Can you work these out from the model? Positions are in its coordinate system, mm. Face numbers are marked on the shaded views. A direction names the side the tool comes from. Coordinates: 2 decimals unless noted, no trailing zeros. Order: outer loops, then holes, each group sorted by start corner. A loop starts at its lowest first (then second) coordinate and runs counter-clockwise, first axis right, second up. Notation, with made-up numbers: (20.25, -25) -> (37.25, -25) arc R12 ccw to (37.25, -20) -> close; hole circle Ø6 at (-6, 37.5). An arc over 180 degrees is marked (long way). Return JSON: item names as keys, results as strings. Group by question number.
1) If we section it at D-D, the plane y = 0: Please give me the cut outline in (x, z).
2) For the marked faces 4, 5 and 6, which set-ups out of +Z, -Z, +X, -X, +Y, -Y let a thin tool reach every point of the face, with its end or its side?
3) If we section it at C-C, the plane z = -19.5: Please give me the cut outline in (x, y), then the cut area to 3 significant figures.
4) If we section it at A-A, the plane y = 23.5: Please give me the cut outline in (x, z).
5) Thinking about a two-plate mould opening in Z: for the marked faces 1, 2 and 3, which applies, +Z half, -Z half, draft (parallel to the pull), parting line (faces both ways), or undercut?
6) If we section it at B-B, the plane x = 0: Please give me the cut outline in (y, z), then the cut area to 3 significant figures.
7) If I drill on probe 1 along X at (y, z) = (22, -8); probe 2 along Y at (x, z) = (0, 1.7); probe 3 along Z at (x, y) = (0.25, 7.5), over which ranges is the centre line in solid material (lowest first)? Write a range as from..to.
8) For pin 1 (5.5 mm diameter, centred on y = 41.7, z = -19.5, fed in from -X); pin 2 (5 mm diameter, centred on x = 0, y = 0, fed in from -Z); pin 3 (4 mm diameter, centred on x = -3.5, z = -7, fed in from -Y), each with a flat end and sliding along its axis, tell me the tip position at first contact or that it passes through.
from build123d import *
from OCP.BRepFilletAPI import BRepFilletAPI_MakeChamfer

# Parameters (mm, degrees)
SKETCH1_W           = 18
SKETCH1_H           = 25.4
SKETCH1_R           = 3.25
BOSS_EXTRUDE1_DEPTH = 6
SKETCH2_W           = 18
SKETCH2_H           = 37.5
BOSS_EXTRUDE2_DEPTH = 6
SKETCH3_W           = 5.95
SKETCH3_H           = 37.5
BOSS_EXTRUDE3_DEPTH = 35
SKETCH4_R           = 2.15
CUT_EXTRUDE1_DEPTH  = 65.806944072
CUT_EXTRUDE2_REACH  = 66.807
SKETCH5_R           = 2.95
FILLET1_R           = 10
FILLET2_R           = 6
CHAMFER1_SIZE       = 1
CHAMFER1_SIZE2      = 1.732050808
CHAMFER2_SIZE       = 1
CHAMFER2_SIZE2      = 1.732050808
FILLET3_R           = 1


with BuildPart() as part:
    # Sketch1 → Boss-Extrude1 (new body)
    with BuildSketch(Plane.XY):
        Rectangle(SKETCH1_W, SKETCH1_H)
        Circle(SKETCH1_R, mode=Mode.SUBTRACT)
    boss_extrude1 = extrude(amount=BOSS_EXTRUDE1_DEPTH)

    # Sketch2 → Boss-Extrude2 (add)
    with BuildSketch(Plane(origin=(0, 12.7, 0), x_dir=(1, 0, 0), z_dir=(0, 1, 0))):
        with Locations((0, 12.75)):
            Rectangle(SKETCH2_W, SKETCH2_H)
    extrude(amount=BOSS_EXTRUDE2_DEPTH)

    # Mirror1: Boss-Extrude1 across plane
    add(boss_extrude1.mirror(Plane.XY.offset(-12.75)))

    # Sketch3 → Boss-Extrude3 (add)
    with BuildSketch(Plane(origin=(0, 18.7, 0), x_dir=(1, 0, 0), z_dir=(0, 1, 0))):
        with Locations((6.025, 12.75)):
            Rectangle(SKETCH3_W, SKETCH3_H)
    boss_extrude3 = extrude(amount=BOSS_EXTRUDE3_DEPTH)

    # Mirror2: Boss-Extrude3 across plane
    add(boss_extrude3.mirror(Plane(origin=(0, 0, 0), x_dir=(0, 0, 1), z_dir=(1, 0, 0))))

    # Sketch4 → Cut-Extrude1 (cut, through all)
    with BuildSketch(Plane(origin=(9, 0, 0), x_dir=(0, 0, -1), z_dir=(1, 0, 0))):
        with Locations((19.5, 41.7)):
            Circle(SKETCH4_R)
    extrude(amount=-CUT_EXTRUDE1_DEPTH, mode=Mode.SUBTRACT)

    # Sketch5 → Cut-Extrude2 (cut, up to next)
    with BuildSketch(Plane.ZY.offset(9), mode=Mode.PRIVATE) as cut_extrude2_sk1:
        with Locations((-19.5, 41.7)):
            Circle(SKETCH5_R)
    cut_extrude2_tool1 = extrude(cut_extrude2_sk1.sketch, amount=-CUT_EXTRUDE2_REACH, mode=Mode.PRIVATE) & part.part
    add(cut_extrude2_tool1.solids().sort_by_distance((-9, 41.7, -19.5))[0], mode=Mode.SUBTRACT)

    # Fillet1
    fillet1_edges = [part.edges().sort_by_distance(p)[0] for p in [
        (6.025, 53.7, -31.5),
        (6.025, 53.7, 6),
        (-6.025, 53.7, 6),
        (-6.025, 53.7, -31.5),
    ]]
    fillet(fillet1_edges, radius=FILLET1_R)

    # Fillet2
    fillet2_edges = [part.edges().sort_by_distance(p)[0] for p in [
        (9, -12.7, -28.5),
        (-9, -12.7, -28.5),
        (9, -12.7, 3),
        (-9, -12.7, 3),
    ]]
    fillet(fillet2_edges, radius=FILLET2_R)

    # Chamfer1: one chamfer whose edges measure the first distance from different faces: ONE call of the kernel's chamfer builder (chamfer() names one face for all edges)
    chamfer1_edges_1 = [part.edges().sort_by_distance(p)[0] for p in [
        (-3.05, 31.2, -31.5),
        (3.05, 31.2, -31.5),
    ]]
    chamfer1_side_1 = [part.faces().sort_by_distance(p)[0] for p in [
        (0, 13.700522402, -31.5),
    ]]
    chamfer1_edges_2 = [part.edges().sort_by_distance(p)[0] for p in [
        (-3.05, 53.7, -12.75),
    ]]
    chamfer1_side_2 = [part.faces().sort_by_distance(p)[0] for p in [
        (-6.025, 53.7, -12.75),
    ]]
    chamfer1_edges_3 = [part.edges().sort_by_distance(p)[0] for p in [
        (-3.05, 31.2, 6),
        (3.05, 31.2, 6),
    ]]
    chamfer1_side_3 = [part.faces().sort_by_distance(p)[0] for p in [
        (0, 13.700522402, 6),
    ]]
    chamfer1_edges_4 = [part.edges().sort_by_distance(p)[0] for p in [
        (-3.05, 50.771067812, 3.071067812),
    ]]
    chamfer1_side_4 = [part.faces().sort_by_distance(p)[0] for p in [
        (-6.025, 50.771067812, 3.071067812),
    ]]
    chamfer1_edges_5 = [part.edges().sort_by_distance(p)[0] for p in [
        (-3.05, 50.771067812, -28.571067812),
    ]]
    chamfer1_side_5 = [part.faces().sort_by_distance(p)[0] for p in [
        (-6.025, 50.771067812, -28.571067812),
    ]]
    chamfer1_edges_6 = [part.edges().sort_by_distance(p)[0] for p in [
        (3.05, 53.7, -12.75),
    ]]
    chamfer1_side_6 = [part.faces().sort_by_distance(p)[0] for p in [
        (6.025, 53.7, -12.75),
    ]]
    chamfer1_edges_7 = [part.edges().sort_by_distance(p)[0] for p in [
        (3.05, 50.771067812, 3.071067812),
    ]]
    chamfer1_side_7 = [part.faces().sort_by_distance(p)[0] for p in [
        (6.025, 50.771067812, 3.071067812),
    ]]
    chamfer1_edges_8 = [part.edges().sort_by_distance(p)[0] for p in [
        (3.05, 50.771067812, -28.571067812),
    ]]
    chamfer1_side_8 = [part.faces().sort_by_distance(p)[0] for p in [
        (6.025, 50.771067812, -28.571067812),
    ]]
    chamfer1 = BRepFilletAPI_MakeChamfer(part.part.solid().wrapped)
    for e in chamfer1_edges_1:
        chamfer1.Add(CHAMFER1_SIZE, CHAMFER1_SIZE2, e.wrapped, chamfer1_side_1[0].wrapped)  # the first distance lies on this face
    for e in chamfer1_edges_2:
        chamfer1.Add(CHAMFER1_SIZE, CHAMFER1_SIZE2, e.wrapped, chamfer1_side_2[0].wrapped)  # the first distance lies on this face
    for e in chamfer1_edges_3:
        chamfer1.Add(CHAMFER1_SIZE, CHAMFER1_SIZE2, e.wrapped, chamfer1_side_3[0].wrapped)  # the first distance lies on this face
    for e in chamfer1_edges_4:
        chamfer1.Add(CHAMFER1_SIZE, CHAMFER1_SIZE2, e.wrapped, chamfer1_side_4[0].wrapped)  # the first distance lies on this face
    for e in chamfer1_edges_5:
        chamfer1.Add(CHAMFER1_SIZE, CHAMFER1_SIZE2, e.wrapped, chamfer1_side_5[0].wrapped)  # the first distance lies on this face
    for e in chamfer1_edges_6:
        chamfer1.Add(CHAMFER1_SIZE, CHAMFER1_SIZE2, e.wrapped, chamfer1_side_6[0].wrapped)  # the first distance lies on this face
    for e in chamfer1_edges_7:
        chamfer1.Add(CHAMFER1_SIZE, CHAMFER1_SIZE2, e.wrapped, chamfer1_side_7[0].wrapped)  # the first distance lies on this face
    for e in chamfer1_edges_8:
        chamfer1.Add(CHAMFER1_SIZE, CHAMFER1_SIZE2, e.wrapped, chamfer1_side_8[0].wrapped)  # the first distance lies on this face
    add(Compound.cast(chamfer1.Shape()), mode=Mode.REPLACE)

    # Chamfer2: one chamfer whose edges measure the first distance from different faces: ONE call of the kernel's chamfer builder (chamfer() names one face for all edges)
    chamfer2_edges_1 = [part.edges().sort_by_distance(p)[0] for p in [
        (0, -12.7, -31.5),
        (7.242640687, -10.942640687, -31.5),
        (-7.242640687, -10.942640687, -31.5),
        (9, 18.5, -31.5),
        (-9, 18.5, -31.5),
    ]]
    chamfer2_side_1 = [part.faces().sort_by_distance(p)[0] for p in [
        (0, 12.555366953, -31.5),
    ]]
    chamfer2_edges_2 = [part.edges().sort_by_distance(p)[0] for p in [
        (9, 18.5, 6),
        (0, -12.7, 6),
        (7.242640687, -10.942640687, 6),
        (-7.242640687, -10.942640687, 6),
        (-9, 18.5, 6),
    ]]
    chamfer2_side_2 = [part.faces().sort_by_distance(p)[0] for p in [
        (0, 12.555366953, 6),
    ]]
    chamfer2_edges_3 = [part.edges().sort_by_distance(p)[0] for p in [
        (-9, 53.7, -12.75),
    ]]
    chamfer2_side_3 = [part.faces().sort_by_distance(p)[0] for p in [
        (-6.525, 53.7, -12.75),
    ]]
    chamfer2_edges_4 = [part.edges().sort_by_distance(p)[0] for p in [
        (-9, 50.771067812, 3.071067812),
    ]]
    chamfer2_side_4 = [part.faces().sort_by_distance(p)[0] for p in [
        (-6.525, 50.771067812, 3.071067812),
    ]]
    chamfer2_edges_5 = [part.edges().sort_by_distance(p)[0] for p in [
        (-9, 50.771067812, -28.571067812),
    ]]
    chamfer2_side_5 = [part.faces().sort_by_distance(p)[0] for p in [
        (-6.525, 50.771067812, -28.571067812),
    ]]
    chamfer2_edges_6 = [part.edges().sort_by_distance(p)[0] for p in [
        (9, 53.7, -12.75),
    ]]
    chamfer2_side_6 = [part.faces().sort_by_distance(p)[0] for p in [
        (6.525, 53.7, -12.75),
    ]]
    chamfer2_edges_7 = [part.edges().sort_by_distance(p)[0] for p in [
        (9, 50.771067812, 3.071067812),
    ]]
    chamfer2_side_7 = [part.faces().sort_by_distance(p)[0] for p in [
        (6.525, 50.771067812, 3.071067812),
    ]]
    chamfer2_edges_8 = [part.edges().sort_by_distance(p)[0] for p in [
        (9, 50.771067812, -28.571067812),
    ]]
    chamfer2_side_8 = [part.faces().sort_by_distance(p)[0] for p in [
        (6.525, 50.771067812, -28.571067812),
    ]]
    chamfer2 = BRepFilletAPI_MakeChamfer(part.part.solid().wrapped)
    for e in chamfer2_edges_1:
        chamfer2.Add(CHAMFER2_SIZE, CHAMFER2_SIZE2, e.wrapped, chamfer2_side_1[0].wrapped)  # the first distance lies on this face
    for e in chamfer2_edges_2:
        chamfer2.Add(CHAMFER2_SIZE, CHAMFER2_SIZE2, e.wrapped, chamfer2_side_2[0].wrapped)  # the first distance lies on this face
    for e in chamfer2_edges_3:
        chamfer2.Add(CHAMFER2_SIZE, CHAMFER2_SIZE2, e.wrapped, chamfer2_side_3[0].wrapped)  # the first distance lies on this face
    for e in chamfer2_edges_4:
        chamfer2.Add(CHAMFER2_SIZE, CHAMFER2_SIZE2, e.wrapped, chamfer2_side_4[0].wrapped)  # the first distance lies on this face
    for e in chamfer2_edges_5:
        chamfer2.Add(CHAMFER2_SIZE, CHAMFER2_SIZE2, e.wrapped, chamfer2_side_5[0].wrapped)  # the first distance lies on this face
    for e in chamfer2_edges_6:
        chamfer2.Add(CHAMFER2_SIZE, CHAMFER2_SIZE2, e.wrapped, chamfer2_side_6[0].wrapped)  # the first distance lies on this face
    for e in chamfer2_edges_7:
        chamfer2.Add(CHAMFER2_SIZE, CHAMFER2_SIZE2, e.wrapped, chamfer2_side_7[0].wrapped)  # the first distance lies on this face
    for e in chamfer2_edges_8:
        chamfer2.Add(CHAMFER2_SIZE, CHAMFER2_SIZE2, e.wrapped, chamfer2_side_8[0].wrapped)  # the first distance lies on this face
    add(Compound.cast(chamfer2.Shape()), mode=Mode.REPLACE)

    # Fillet3
    fillet3_edges = [part.edges().sort_by_distance(p)[0] for p in [
        (9, 3, -25.5),
        (0, -12.7, -25.5),
        (7.242640687, -10.942640687, -25.5),
        (-7.242640687, -10.942640687, -25.5),
        (9, 3, 0),
        (0, -12.7, 0),
        (7.242640687, -10.942640687, 0),
        (-7.242640687, -10.942640687, 0),
        (9, 12.7, -12.75),
        (-9, 12.7, -12.75),
        (-9, 3, -25.5),
        (-9, 3, 0),
    ]]
    fillet(fillet3_edges, radius=FILLET3_R)


solid = part.part
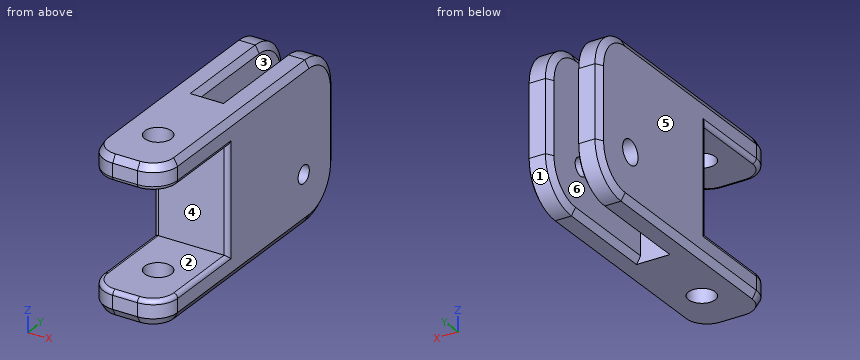
Result sheet:
{
 "1": {"outline": "(-9, -29.77) -> (-8, -31.5) -> (-3.25, -31.5) -> (-3.25, -25.5) -> (-8, -25.5) arc R1 ccw to (-9, -26.5) -> close; (-9, 1) arc R1 ccw to (-8, 0) -> (-3.25, 0) -> (-3.25, 6) -> (-8, 6) -> (-9, 4.27) -> close; (3.25, -31.5) -> (8, -31.5) -> (9, -29.77) -> (9, -26.5) arc R1 ccw to (8, -25.5) -> (3.25, -25.5) -> close; (3.25, 0) -> (8, 0) arc R1 ccw to (9, 1) -> (9, 4.27) -> (8, 6) -> (3.25, 6) -> close"},
 "2": {"face 4": "+X, -X, -Y", "face 5": "+Z, -Z, -X, +Y, -Y", "face 6": "+Z, -Z, +Y"},
 "3": {"outline": "(-9, 13.7) arc R1 ccw to (-8, 12.7) -> (8, 12.7) arc R1 ccw to (9, 13.7) -> (9, 39.55) -> (3.05, 39.55) -> (3.05, 18.7) -> (-3.05, 18.7) -> (-3.05, 38.75) -> (-9, 38.75) -> close; (-9, 44.65) -> (-3.05, 44.65) -> (-3.05, 51.97) -> (-4.05, 53.7) -> (-8, 53.7) -> (-9, 51.97) -> close; (3.05, 43.85) -> (9, 43.85) -> (9, 51.97) -> (8, 53.7) -> (4.05, 53.7) -> (3.05, 51.97) -> close", "area": "460 mm2"},
 "4": {"outline": "(-9, -29.77) -> (-8, -31.5) -> (-4.05, -31.5) -> (-3.05, -29.77) -> (-3.05, 4.27) -> (-4.05, 6) -> (-8, 6) -> (-9, 4.27) -> close; (3.05, -29.77) -> (4.05, -31.5) -> (8, -31.5) -> (9, -29.77) -> (9, 4.27) -> (8, 6) -> (4.05, 6) -> (3.05, 4.27) -> close"},
 "5": {"face 1": "-Z half", "face 2": "undercut", "face 3": "draft"},
 "6": {"outline": "(-12.7, -29.77) -> (-11.7, -31.5) -> (-3.25, -31.5) -> (-3.25, -25.5) -> (-11.7, -25.5) arc R1 ccw to (-12.7, -26.5) -> close; (-12.7, 1) arc R1 ccw to (-11.7, 0) -> (-3.25, 0) -> (-3.25, 6) -> (-11.7, 6) -> (-12.7, 4.27) -> close; (3.25, -31.5) -> (18.7, -31.5) -> (18.7, 6) -> (3.25, 6) -> (3.25, 0) -> (12.7, 0) -> (12.7, -25.5) -> (3.25, -25.5) -> close", "area": "450 mm2"},
 "7": {"probe 1": "x = -9..-3.05, 3.05..9", "probe 2": "y = -12.7..-3.25, 3.25..18.7", "probe 3": "z = -31.5..-25.5, 0..6"},
 "8": {"pin 1": "stops at x = 3.05", "pin 2": "passes through", "pin 3": "stops at y = 12.7"}
}
